Build history of the part. All positions in model axes, mm. A direction names the side the tool comes from. Give positions to 0.01 mm unless a question says otherwise; leave off trailing zeros. Write each loop counter-clockwise with the first axis right and the second up, starting at its lowest first coordinate (ties: lowest second). Pieces come first, ordered by that corner, then holes. Notation, with made-up numbers: (-15, -35) -> (-4, -35) arc R29 cw to (-4, -13) -> close; hole circle Ø4 at (19.25, -24). An arc over 180 degrees is marked (long way). Write item = value, one per line. Start each with the question number.
Q1. Saw through at A-A, the plane z = 0. List the corners of the cut face in (x, y) (3 decimals), then the cut area to 3 significant figures.
Q2. Saw through at D-D, the plane x = 1. List the corners of the cut face in (y, z) (3 decimals), then the cut area to 3 significant figures.
Q3. Wall check: line 1 (X direction, y = -0.25, z = -5); line 2 (Y direction, x = 1.75, z = 0.75); line 3 (X direction, y = -2.75, z = 1.75). Give the ranges that are in metal, low to high.
Q4. Saw through at B-B, the plane y = 0. List the corners of the cut face in (x, z), then the cut area to 3 significant figures.
Q5. Drop flat-ended pins along their axis: P1, Ø3, axis at x = 1.5, z = 5.5, coming from the +Y side; P2, Ø3, axis at y = 3.5, z = -1, coming from the +X side; P3, Ø4, axis at x = 8.5, z = -4.5, coming from the +Y side; P4, Ø1.5, axis at x = 9.5, z = 0, coming from the +Y side. Give the stop position or say it passes through.
Q6. Saw through at C-C, the plane x = 3.5. List the corners of the cut face in (y, z), then the cut area to 3 significant figures.
Q7. Tool access for faces 5 (the face through (1, 0.6, 0)), 6 (the face through (2.022, 2.103, -6.677)): list every direction of +Z, -Z, +X, -X, +Y, -Y with a clear straight run to the whole face (end or side of a thin tool).
Q8. Mould opens along Y. For faces 1 (the face through (1.4, 0, 0)), 2 (the face through (2.8, 2, 2)), 3 (the face through (6.663, 0.601, -1.908)), 4 (the face through (1, -0.6, 0)) say: pulls with the +Y half, pulls with the -Y half, needs draft (parallel to the pull), parting line crosses it, or undercut.
from build123d import *

# Parameters (mm, degrees)
SKETCH1_R       = 7
BASEHEAD_DEPTH  = 2.8
SKETCH2_R       = 2
BASEBODY_DEPTH  = 8
SLOT_DEPTH      = 15.650597257
SLOT_DEPTH_BACK = 15.650597257
SKETCH3_W       = 1.4
SKETCH3_H       = 1.2
HEADFILLET_R    = 0.2


with BuildPart() as part:
    # Sketch1 → BaseHead (new body)
    with BuildSketch(Plane(origin=(0, 0, 0), x_dir=(0, 0, -1), z_dir=(1, 0, 0))):
        Circle(SKETCH1_R)
    extrude(amount=BASEHEAD_DEPTH)

    # Sketch2 → BaseBody (add)
    with BuildSketch(Plane(origin=(2.8, 0.067556317, 0.30150137), x_dir=(0, 0, -1), z_dir=(1, 0, 0))):
        with Locations((0.30150137, -0.067556317)):
            Circle(SKETCH2_R)
    extrude(amount=BASEBODY_DEPTH)

    # Sketch3 → Slot (cut, two sides: drawn at the far end of the back side and taken through both)
    with BuildSketch(Plane.XY.offset(-SLOT_DEPTH_BACK)):
        with Locations((0.7, 0)):
            Rectangle(SKETCH3_W, SKETCH3_H)
    extrude(amount=SLOT_DEPTH + SLOT_DEPTH_BACK, mode=Mode.SUBTRACT)

    # Sketch4 → BaseTop (revolve, cut)
    with BuildSketch(Plane(origin=(-5.763764327, 3.913764327, 0), x_dir=(0, -1, 0), z_dir=(0, 0, 1))):
        with BuildLine():
            Line((1.913764327, 18.563764327), (1.913764327, 16.194443059))
            ThreePointArc((1.913764327, 16.194443059), (2.896857473, 16.470660045), (3.913764327, 16.563764327))
            Line((3.913764327, 16.563764327), (3.913764327, 18.563764327))
            Line((3.913764327, 18.563764327), (1.913764327, 18.563764327))
        make_face()
        with BuildLine():
            Line((-3.086235673, 3.763764327), (3.913764327, 3.763764327))
            Line((3.913764327, 3.763764327), (3.913764327, 5.763764327))
            ThreePointArc((3.913764327, 5.763764327), (0.357072037, 6.08255654), (-3.086235673, 7.028770332))
            Line((-3.086235673, 7.028770332), (-3.086235673, 3.763764327))
        make_face()
    revolve(axis=Axis((9.335097479, 0, 0), (-1, 0, 0)), mode=Mode.SUBTRACT)

    # HeadFillet
    headfillet_edges = [part.edges().sort_by_distance(p)[0] for p in [
        (2.8, 0, 2),
    ]]
    fillet(headfillet_edges, radius=HEADFILLET_R)


solid = part.part
Report:
q1.outline = (0.009, -0.6) arc R20 ccw to (1.265, -7) -> (2.8, -7) -> (2.8, -2.2) arc R0.2 cw to (3, -2) -> (10.431, -2) arc R5.6 ccw to (10.431, 2) -> (3, 2) arc R0.2 cw to (2.8, 2.2) -> (2.8, 7) -> (1.265, 7) arc R20 ccw to (0.009, 0.6) -> (1.4, 0.6) -> (1.4, -0.6) -> close
q1.area = 63.2 mm2
q2.outline = (-0.6, -6.216) -> (-0.6, 6.216) arc R6.245 ccw to start; (0.6, -6.216) arc R6.245 ccw to (0.6, 6.216) -> close
q2.area = 108 mm2
q3.line_1 = 1.4 to 2.8
q3.line_2 = -6.96 to 6.96
q3.line_3 = 0.27 to 2.8
q4.outline = (1.4, -7) -> (2.8, -7) -> (2.8, -2.2) arc R0.2 cw to (3, -2) -> (10.43, -2) arc R5.6 ccw to (10.43, 2) -> (3, 2) arc R0.2 cw to (2.8, 2.2) -> (2.8, 7) -> (1.4, 7) -> close
q4.area = 51.1 mm2
q5.P1 = 5.74
q5.P2 = 2.81
q5.P3 = through
q5.P4 = 2
q6.outline = circle Ø4 at (0, 0)
q6.area = 12.6 mm2
q7.face_5 = +Z, -Z, -X
q7.face_6 = +X, -X
q8.face_1 = undercut
q8.face_2 = needs draft
q8.face_3 = parting line crosses it
q8.face_4 = undercut
